from build123d import *

# Parameters (mm, degrees)
SKETCH1_R           = 48.26
BOSS_EXTRUDE1_DEPTH = 38.1
SKETCH3_R           = 34.844372605
CUT_EXTRUDE2_DEPTH  = 50.8
FILLET1_R           = 2.54


with BuildPart() as part:
    # Sketch1 → Boss-Extrude1 (new, symmetric)
    with BuildSketch(Plane(origin=(0, 0, 0), x_dir=(1, 0, 0), z_dir=(0, 1, 0))):
        with Locations(Location((0, 0, 0), (0, 0, 90))):
            Circle(SKETCH1_R)
    extrude(amount=BOSS_EXTRUDE1_DEPTH, both=True)

    # Sketch3 → Cut-Extrude2 (cut)
    with BuildSketch(Plane(origin=(0, 38.1, 0), x_dir=(1, 0, 0), z_dir=(0, 1, 0))):
        with Locations(Location((0, 0, 0), (0, 0, 270))):
            Circle(SKETCH3_R)
    extrude(amount=-CUT_EXTRUDE2_DEPTH, mode=Mode.SUBTRACT)

    # Fillet1
    fillet1_edges = [part.edges().sort_by_distance(p)[0] for p in [
        (0, -38.1, 48.26),
        (0, 38.1, 48.26),
        (0, 38.1, -34.844372605),
    ]]
    fillet(fillet1_edges, radius=FILLET1_R)


solid = part.part
Input: part model. Units: mm. Frame: model coordinates. A direction names the side the tool comes from. Round coordinates to 2 decimals unless told otherwise and drop trailing zeros. Loops run counter-clockwise (first coordinate to the right, second up) from the corner with the lowest first, then second, coordinate; pieces in that order, holes last. Notation, with made-up numbers: M 29.5,-17.5 L 35.5,-17.5 A26 cw 35.5,17.5 Z; hole C -21,60 d10. An arc over 180 degrees is marked long. Answer as CSV lines item,"result". Start each with the question number.
(1) First-contact query: pin 1 (3 mm diameter, centred on x = -30, y = 25.5, fed in from -Z); pin 2 (6 mm diameter, centred on x = -4, z = 4, fed in from +Y); pin 3 (12 mm diameter, centred on y = 18, z = 4.5, fed in from -X). Flat tips, straight axial feed; report the tip coordinate or a pass-through.
(2) Reachability of faces 1 (the flat face through (34, 38.1, 17)), 2 (the flat face through (0, -12.7, 0)) from +Z, -Z, +X, -X, +Y, -Y: full face, straight path, thin tool, end or side. Return the list, or none.
(3) Section A-A, the plane z = 0. Output: boundary loops of the cut face in (x, y).
(4) Draft query along Z for faces 3 (the cylindrical face through (-34.016, 11.768, -7.554)), 4 (the cylindrical face through (-14.5, 0.5, -46.03)), 5 (the flat face through (-1, -38.1, 1)). Return one class per face: released by +Z, released by -Z, zero draft, split by the parting line, or undercut.
(5) Line query: line 1 (X direction, y = 17, z = 0); line 2 (Y direction, x = -31.5, z = -14); line 3 (X direction, y = 12.5, z = -4). Output: solid intervals per line, ascending. Write a range as [from, to].
(6) Section D-D, the plane y = -20.5. Output: boundary loops of the cut face in (x, z), plus the area to 3 significant figures.
(7) Section C-C, the plane x = 0. Output: boundary loops of the cut face in (y, z).
(8) Section B-B, the plane y = -6. Output: boundary loops of the cut face in (x, z), plus the area to 3 significant figures.
Values found:
1,pin 1,"stops at z = -38.95"
1,pin 2,"stops at y = -12.7"
1,pin 3,"stops at x = -48.26"
2,face 1,"+Z, -Z, +X, -X, +Y"
2,face 2,"+Y"
3,outline,"M -48.26,-35.56 A2.54 ccw -45.72,-38.1 L 45.72,-38.1 A2.54 ccw 48.26,-35.56 L 48.26,35.56 A2.54 ccw 45.72,38.1 L 37.38,38.1 A2.54 ccw 34.84,35.56 L 34.84,-12.7 L -34.84,-12.7 L -34.84,35.56 A2.54 ccw -37.38,38.1 L -45.72,38.1 A2.54 ccw -48.26,35.56 Z"
4,face 3,"undercut"
4,face 4,"split by the parting line"
4,face 5,"zero draft"
5,line 1,"x = [-48.26, -34.84], [34.84, 48.26]"
5,line 2,"y = [-38.1, -12.7]"
5,line 3,"x = [-48.09, -34.61], [34.61, 48.09]"
6,outline,"C 0,0 d96.52"
6,area,"7,320 mm²"
7,outline,"M -38.1,-45.72 A2.54 ccw -35.56,-48.26 L 35.56,-48.26 A2.54 ccw 38.1,-45.72 L 38.1,-37.38 A2.54 ccw 35.56,-34.84 L -12.7,-34.84 L -12.7,34.84 L 35.56,34.84 A2.54 ccw 38.1,37.38 L 38.1,45.72 A2.54 ccw 35.56,48.26 L -35.56,48.26 A2.54 ccw -38.1,45.72 Z"
8,outline,"C 0,0 d96.52; hole C 0,0 d69.69"
8,area,"3,500 mm²"
